Geometry: final body of the model. Coordinates: model frame, mm. Face numbers are marked on the shaded views. Give positions to 0.01 mm unless a question says otherwise; leave off trailing zeros. Order: outer loops, then holes, each group sorted by start corner. A loop starts at its lowest first (then second) coordinate and runs counter-clockwise, first axis right, second up. Notation, with made-up numbers: (70, 70.25) -> (126, 70.25) arc R30 ccw to (126, 100.25) -> close; hole circle Ø9 at (43, 83.5). An arc over 180 degrees is marked (long way). One line per item, written item: value. Start each with the question number.
```python
from build123d import *

# Parameters (mm, degrees)
BOSS_EXTRUDE1_DEPTH = 4.826


with BuildPart() as part:
    # Sketch1 → Boss-Extrude1 (new body)
    with BuildSketch(Plane.XY):
        with BuildLine():
            ThreePointArc((18.442512073, 8.741762413), (-3.782487927, -13.483237587), (-26.007487927, 8.741762413))
            Line((-26.007487927, 8.741762413), (-26.007487927, 18.211893689))
            ThreePointArc((-26.007487927, 18.211893689), (-9.547899201, -30.280358664), (31.75, 0))
            ThreePointArc((31.75, 0), (28.227754589, 14.534661016), (18.442512073, 25.844462626))
            Line((18.442512073, 25.844462626), (18.442512073, 8.741762413))
        make_face()
    extrude(amount=BOSS_EXTRUDE1_DEPTH)


solid = part.part
```
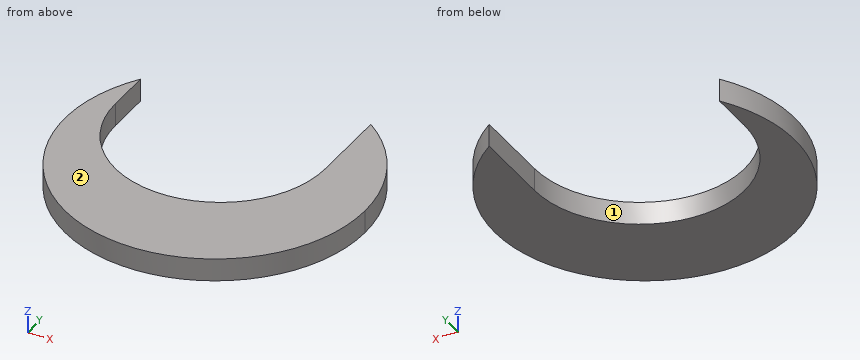
1. Cut plane C-C, the plane x = -7. Return loops of the section in (y, z), then the cut area to 3 significant figures.
2. Draft query along X for the marked faces 1 and 2. Return one class per face: pulls with the +X half, pulls with the -X half, needs draft (parallel to the pull), parting line crosses it, or undercut.
3. Material intervals for L1, parallel to X at y = 16, z = 0.8; L2, parallel to X at y = 17, z = 2.6; L3, parallel to Y at x = -16.5, z = 3, sorted ascending. Write a range as [from, to].
4. Cut plane B-B, the plane z = 2.2. Return loops of the section in (x, y) (3 decimals).
5. Cut plane A-A, the plane y = 13. Return loops of the section in (x, z), then the cut area to 3 significant figures.
6. Cut plane D-D, the plane y = 21. Return loops of the section in (x, z), then the cut area to 3 significant figures.
7. Pin query (flat end, axial travel): P1, Ø2.5, axis at y = 14, z = 3, coming from the +X side; P2, Ø2, axis at x = -22, y = -10, coming from the -Z side; P3, Ø2, axis at y = -25.5, z = 2, coming from the +X side; P4, Ø2.5, axis at y = 17, z = 2.5, coming from the -X side. Return the tip coordinate at first contact, or that it passes through.
Answers follow:
1. outline: (-30.97, 0) -> (-13.25, 0) -> (-13.25, 4.83) -> (-30.97, 4.83) -> close
1. area: 85.5 mm²
2. face 1: undercut
2. face 2: needs draft
3. L1: x = [-27.42, -26.01], [18.44, 27.42]
3. L2: x = [-26.82, -26.01], [18.44, 26.82]
3. L3: y = [-27.13, -9.49]
4. outline: (-26.007, 8.742) -> (-26.007, 18.212) arc R31.75 ccw (long way) to (18.443, 25.844) -> (18.443, 8.742) arc R22.225 cw to start
5. outline: (-28.97, 0) -> (-26.01, 0) -> (-26.01, 4.83) -> (-28.97, 4.83) -> close; (18.44, 0) -> (28.97, 0) -> (28.97, 4.83) -> (18.44, 4.83) -> close
5. area: 65.1 mm²
6. outline: (18.44, 0) -> (23.81, 0) -> (23.81, 4.83) -> (18.44, 4.83) -> close
6. area: 25.9 mm²
7. P1: stops at x = 29.08
7. P2: stops at z = 0
7. P3: stops at x = 20.19
7. P4: stops at x = -27.57
